Geometry: final body of the model. Coordinates: model frame, mm. A direction names the side the tool comes from. Give positions to 0.01 mm unless a question says otherwise; leave off trailing zeros. Write each loop counter-clockwise with the first axis right and the second up, starting at its lowest first coordinate (ties: lowest second). Pieces come first, ordered by that corner, then holes. Notation, with made-up numbers: (80.5, 44.5) -> (104.5, 44.5) arc R31 cw to (104.5, 79.5) -> close; hole circle Ø6 at (-24, -20). An arc over 180 degrees is marked (long way). Answer in a Markdown table with one row per item. Add a question column.
Item 1: Section query C-C on z = 0. Output: boundary loops of the cut face in (x, y), plus the area to 3 significant figures.
Item 2: Section query D-D on x = -8.5. Output: boundary loops of the cut face in (y, z).
Item 3: Material intervals for probe 1 along Y at (x, z) = (-71, 0.5); probe 2 along X at (y, z) = (8, 9.75); probe 3 along Z at (x, y) = (-50, 4.75), sorted ascending. Write a range as from..to.
Item 4: First-contact query: P1, Ø2, axis at y = -4.5, z = 3.5, coming from the -X side; P2, Ø11, axis at x = -40, y = 5.5, coming from the +Z side; P3, Ø2, axis at y = 5, z = 11.5, coming from the -X side; P4, Ø1.5, axis at y = -5, z = 8, coming from the -X side. Flat tips, straight axial feed; report the tip coordinate or a pass-through.
Item 5: Section query A-A on y = -6.25. Output: boundary loops of the cut face in (x, z) (3 decimals).
Item 6: Access query for faces 1 (the flat face through (-37, 5, 7.35)), 2 (the flat face through (-37, 5, -7.5)), 3 (the flat face through (24, 5, 14.72)), 4 (the cylindrical face through (-81.666, -4.93, -4.74)). Directions: +Z, -Z, +X, -X, +Y, -Y. A direction counts if a zero-diameter tool reaches every point of the face in a straight line with its end or side. Return the directions, or none.
Item 7: Section query B-B on y = 1.5. Output: boundary loops of the cut face in (x, z).
```python
from build123d import *

# Parameters (mm, degrees)
EXTRUDE_1_DEPTH        = 10
SKETCH_3_R             = 2.392945251
SKETCH_3_R_2           = 2.39
EXTRUDE_2_DEPTH        = 10
PATTERN_LINEAR_1_COUNT = 4
PATTERN_LINEAR_1_PITCH = 27.05


with BuildPart() as part:
    # 草图1 → 凸台-拉伸1 (new body)
    with BuildSketch(Plane(origin=(0, 0, 0), x_dir=(1, 0, 0), z_dir=(0, 1, 0))):
        Polygon((-88.703690987, 0), (-88.703690987, 7.5), (-83.873690987, 7.5), (-56.823690987, 7.5), (-29.773690987, 7.5), (-2.723690987, 7.5), (12.386309013, 7.5), (12.386309013, 11.82), (36.006309013, 11.82), (36.006309013, -14.72), (12.386309013, -14.72), (12.386309013, -7.35), (-88.703690987, -7.35), align=None)
    extrude(amount=EXTRUDE_1_DEPTH)

    # 草图3 → 凸台-拉伸2 (add)
    with BuildSketch(Plane.XZ):
        with Locations((-83.873690987, 3.675)):
            Circle(SKETCH_3_R)
        with Locations((-83.873690987, -3.825)):
            Circle(SKETCH_3_R_2)
    extrude_2 = extrude(amount=EXTRUDE_2_DEPTH)

    # 阵列(线性)1: 凸台-拉伸2 ×4
    with Locations(*[(i * PATTERN_LINEAR_1_PITCH, 0, 0) for i in range(1, PATTERN_LINEAR_1_COUNT)]):
        add(extrude_2)


solid = part.part
```
Findings below:
| question | item | result |
|---|---|---|
| 1 | outline | (-88.7, 0) -> (36.01, 0) -> (36.01, 10) -> (-88.7, 10) -> close |
| 1 | area | 1,250 mm^2 |
| 2 | outline | (0, -7.5) -> (10, -7.5) -> (10, 7.35) -> (0, 7.35) -> close |
| 3 | probe 1 | y = 0..10 |
| 3 | probe 2 | x = 12.39..36.01 |
| 3 | probe 3 | z = -7.5..7.35 |
| 4 | P1 | stops at x = -86.27 |
| 4 | P2 | stops at z = 7.35 |
| 4 | P3 | stops at x = 12.39 |
| 4 | P4 | passes through |
| 5 | outline | circle Ø4.786 at (-83.874, 3.675); circle Ø4.78 at (-83.874, -3.825); circle Ø4.786 at (-56.824, 3.675); circle Ø4.78 at (-56.824, -3.825); circle Ø4.786 at (-29.774, 3.675); circle Ø4.78 at (-29.774, -3.825); circle Ø4.786 at (-2.724, 3.675); circle Ø4.78 at (-2.724, -3.825) |
| 6 | face 1 | +Z, -X, +Y, -Y |
| 6 | face 2 | -Z, -X, +Y, -Y |
| 6 | face 3 | +Z, +X, -X, +Y, -Y |
| 6 | face 4 | -Y |
| 7 | outline | (-88.7, -7.5) -> (12.39, -7.5) -> (12.39, -11.82) -> (36.01, -11.82) -> (36.01, 14.72) -> (12.39, 14.72) -> (12.39, 7.35) -> (-88.7, 7.35) -> close |
